```python
from build123d import *

# Parameters (mm, degrees)
SKETCH1_R           = 31.75
SKETCH1_R_2         = 30.5054
BOSS_EXTRUDE1_DEPTH = 457.2
SKETCH3_R           = 0.75
CUT_EXTRUDE1_DEPTH  = 460.399570091
CIRPATTERN1_COUNT   = 4


with BuildPart() as part:
    # Sketch1 → Boss-Extrude1 (new body)
    with BuildSketch(Plane.XY):
        Circle(SKETCH1_R)
        Circle(SKETCH1_R_2, mode=Mode.SUBTRACT)
    extrude(amount=BOSS_EXTRUDE1_DEPTH)

    # Sketch3 → Cut-Extrude1 (cut, symmetric)
    with BuildSketch(Plane(origin=(0, 0, 0), x_dir=(1, 0, 0), z_dir=(0, 1, 0))):
        with Locations(Location((0, -381, 0), (0, 0, 270))):
            Circle(SKETCH3_R)
    cut_extrude1 = extrude(amount=CUT_EXTRUDE1_DEPTH, both=True, mode=Mode.SUBTRACT)

    # CirPattern1: Cut-Extrude1 ×4 about axis
    cirpattern1_axis = Axis((0, 0, 457.2), (0, 0, -1))
    for i in range(1, CIRPATTERN1_COUNT):
        add(cut_extrude1.rotate(cirpattern1_axis, i * 360 / CIRPATTERN1_COUNT), mode=Mode.SUBTRACT)


solid = part.part
```
Build history of the part. All positions in model axes, mm. Round coordinates to 2 decimals unless told otherwise and drop trailing zeros. Write each loop counter-clockwise with the first axis right and the second up, starting at its lowest first coordinate (ties: lowest second). Pieces come first, ordered by that corner, then holes.
1) Band-saw the part on B-B, the plane y = -20. List the corners of the cut face in (x, z).
2) Mould opens along Y. For faces 1 (the cylindrical face through (29.097, 9.163, 225.4)), 2 (the flat face through (-11.9, 28.4, 0)), 3 (the cylindrical face through (-6.883, -30.995, 225.4)) say: +Y half, -Y half, draft (parallel to the pull), parting line (faces both ways), or undercut.
3) Pin check, flat tips, straight feed: pin 1 (1.7 mm diameter, centred on y = 0, z = 381, fed in from -X); pin 2 (2 mm diameter, centred on x = -21, y = 19, fed in from -Z); pin 3 (1.5 mm diameter, centred on x = 21.5, z = 184, fed in from +Y); pin 4 (3 mm diameter, centred on y = -16.5, z = 234.5, fed in from -X). Stop position of each tip, or through.
4) Drill centre lines: probe 1 along Y at (x, z) = (-2, 77.5); probe 2 along X at (y, z) = (0, 179); probe 3 along Z at (x, y) = (0, 31.3). Where is each one in solid material? Low to high.
5) Band-saw the part on C-C, the plane z = 38. List the corners of the cut face in (x, y), and give its area (3 significant figures).
6) Band-saw the part on A-A, the plane x = -9. List the corners of the cut face in (y, z).
Ans:
1. outline: (-24.66, 0) - (-23.03, 0) - (-23.03, 457.2) - (-24.66, 457.2) - close; (23.03, 0) - (24.66, 0) - (24.66, 457.2) - (23.03, 457.2) - close
2. face 1: undercut
2. face 2: draft
2. face 3: parting line
3. pin 1: stops at x = -31.75
3. pin 2: passes through
3. pin 3: stops at y = 24.03
3. pin 4: stops at x = -27.98
4. probe 1: y = -31.69 to -30.44, 30.44 to 31.69
4. probe 2: x = -31.75 to -30.51, 30.51 to 31.75
4. probe 3: z = 0 to 380.25, 381.75 to 457.2
5. outline: circle Ø63.5 at (0, 0); hole circle Ø61.01 at (0, 0)
5. area: 243 mm2
6. outline: (-30.45, 0) - (-29.15, 0) - (-29.15, 457.2) - (-30.45, 457.2) - close; (29.15, 0) - (30.45, 0) - (30.45, 457.2) - (29.15, 457.2) - close
